Autodesk Inventor part; units mm, degrees
ref_plane "Work Plane2" through (-53.25, -178, -67.8971) normal (0, -1, 0) x (0.8660254, 0, -0.5)
ref_plane "Work Plane5" through (-46.3218, -178, -67.8971) normal (0, -1, 0) x (0.8660254, 0, -0.5)
ref_plane "YZ Plane" through (0, 0, 0) normal (1, 0, 0) x (0, 1, 0)
ref_plane "Work Plane1" through (14.6553, 0, -25.7817) normal (0, 1, 0) x (-0.8660254, 0, 0.5)
ref_plane "Work Plane2" through (-53.25, -178, -67.8971) normal (0, -1, 0) x (0.8660254, 0, -0.5)
ref_plane "Work Plane3" through (14.6553, 0, -25.7817) normal (0, 1, 0) x (-0.8660254, 0, 0.5)
ref_plane "Work Plane4" through (-55.7811, 0, -1.2811) normal (0, 1, 0) x (0.5, 0, 0.8660254)
sketch "Sketch4" plane through (-55.7811, 0, -1.2811) normal (0, 1, 0) x (0.5, 0, 0.8660254)
  line L0 (3.5, 3.5) -> (-1, 3.5)
  line L1 (-1, 3.5) -> (-1, -0.5)
  line L2 (-1, -0.5) -> (-4.5, -0.5)
  line L3 (-4.5, -0.5) -> (-4.5, -14.5)
  line L4 (-4.5, -14.5) -> (4.5, -0.5)
  line L5 (4.5, -0.5) -> (3.5, -0.5)
  line L6 (3.5, -0.5) -> (3.5, 3.5)
  line L7 (3.5, 3.5) -> (29, 47.6673)
  line L8 (29, 47.6673) -> (3.5, 3.5)
  line L9 (3.5, 1.7679) -> (30, 47.6673)
  line L10 (30, 47.6673) -> (29, 47.6673)
  point P0 (29, 47.6673)
  dimension "d10" = 1
ref_plane "Work Plane5" through (-46.3218, -178, -67.8971) normal (0, -1, 0) x (0.8660254, 0, -0.5)
extrude "Extrusion2" add sketch "Sketch4" against normal up to surface (178 mm away) contours L7 L10 L9 L6
sketch "Sketch5" plane through (-52.5, 0, 0.866) normal (0, 0, 1) x (1, 0, 0)
  circle A0 centre (30.6045, -58.5) radius 2.3
  circle A1 centre (45.2015, -58.5) radius 2.3
  circle A2 centre (30.6045, -119.5) radius 2.3
  circle A3 centre (45.2015, -119.5) radius 2.3
  circle A4 centre (48, -3) radius 2
  circle A5 centre (19.3979, -3) radius 2
  circle A6 centre (48, -175) radius 2
  circle A7 centre (19.3979, -175) radius 2
  point P0 (52.5, 0)
hole "Hole2" at (-7.2985, -58.5, 0.866) at (-21.8955, -58.5, 0.866) at (-7.2985, -119.5, 0.866) at (-21.8955, -119.5, 0.866) at (-4.5, -3, 0.866) at (-33.1021, -3, 0.866) at (-4.5, -175, 0.866) at (-33.1021, -175, 0.866) direction (0, 0, -1) diameter 3.6 end through all countersink diameter 6.5 countersink angle 90
properties part number "frobt" material "Nylon 6/6"
Geometry: final body of the model. Coordinates: model frame, mm. Give positions to 0.01 mm unless a question says otherwise; leave off trailing zeros. Write each loop counter-clockwise with the first axis right and the second up, starting at its lowest first coordinate (ties: lowest second). Pieces come first, ordered by that corner, then holes.
1. Section query C-C, the plane y = -49. Return loops of the section in (x, z), then the cut area to 3 significant figures.
2. Line query: probe 1 along X at (y, z) = (-61, 0.6); probe 2 along Y at (x, z) = (-4, 0.15); probe 3 along Y at (x, z) = (-5, 0.7). Output: solid intervals per line, ascending.
3. Section query B-B, the plane z = 0.2. Count the separate pieces of the cut face and the enclosed holes in it, then the cut area to 3 significant figures.
4. Section query A-A, the plane y = -175. Return loops of the section in (x, z), then the cut area to 3 significant figures.
5. Draft query along Y for faces 1 (the conical face through (-3.74, -5.42, 0.15)), 2 (the flat face through (-26, -88, 0)). Return one class per face: released by +Y, released by -Y, zero draft, split by the parting line, or undercut.
Computed:
1. outline: (-52.5, 0.87) - (-51, 0) - (0, 0) - (0.5, 0.87) - close
1. area: 45.0 mm2
2. probe 1: x = -52.04 to -23.52, -20.27 to -8.93, -5.67 to 0.35
2. probe 2: y = -178 to -177.48, -172.52 to -5.48, -0.52 to 0
2. probe 3: y = -171.96 to -121.56, -117.44 to -60.56, -56.44 to -6.04
3. separate pieces: 1
3. enclosed holes: 8
3. area: 8,990 mm2
4. outline: (-52.5, 0.87) - (-51, 0) - (-35.49, 0) - (-36.35, 0.87) - close; (-30.72, 0) - (-6.88, 0) - (-7.75, 0.87) - (-29.85, 0.87) - close; (-2.12, 0) - (0, 0) - (0.5, 0.87) - (-1.25, 0.87) - close
4. area: 35.3 mm2
5. face 1: undercut
5. face 2: zero draft
